from build123d import *

# Parameters (mm, degrees)
EXTRUDE_2_DEPTH     = 34.78
CUT_EXTRUDE_1_REACH = 62.522
SKETCH_2_W          = 20
SKETCH_2_H          = 20
CHAMFER_1_SIZE      = 1
CUT_EXTRUDE_START   = -34.54
SKETCH_3_R          = 2
CUT_EXTRUDE_2_DEPTH = 34.54
SKETCH_4_R          = 2
CUT_EXTRUDE_3_DEPTH = 5
EXTRUDE_START       = -2
EXTRUDE_3_DEPTH     = 5


with BuildPart() as part:
    # 草图1 → 凸台-拉伸2 (new body)
    with BuildSketch(Plane.XY):
        Polygon((0, 0), (0, 35.5), (5, 35.5), (5, 5), (29.54, 5), (29.54, 35.5), (34.54, 35.5), (34.54, 0), align=None)
    extrude(amount=EXTRUDE_2_DEPTH)

    # 切除-拉伸1: up to this face of the body (flat: up to its plane)
    cut_extrude_1_end = Plane(part.part.faces().sort_by_distance((0, 17.75, 17.39))[0])
    # 草图2 → 切除-拉伸1 (cut, up to the picked face)
    with BuildSketch(Plane(origin=(34.54, 0, 0), x_dir=(0, 0, -1), z_dir=(1, 0, 0)), mode=Mode.PRIVATE) as cut_extrude_1_sk1:
        with Locations((-17.28, 15)):
            Rectangle(SKETCH_2_W, SKETCH_2_H)
    cut_extrude_1_tool1 = split(extrude(cut_extrude_1_sk1.sketch, amount=-CUT_EXTRUDE_1_REACH, mode=Mode.PRIVATE), bisect_by=cut_extrude_1_end, keep=Keep.BOTH, mode=Mode.PRIVATE)
    add(cut_extrude_1_tool1.solids().sort_by(Axis((34.54, 15, 17.28), (-1, 0, 0)))[0], mode=Mode.SUBTRACT)

    # 倒角1
    chamfer_1_edges = [part.edges().sort_by_distance(p)[0] for p in [
        (34.54, 17.75, 0),
        (17.27, 0, 0),
        (0, 0, 17.39),
        (34.54, 35.5, 17.39),
        (34.54, 0, 17.39),
        (0, 17.75, 34.78),
        (17.27, 0, 34.78),
        (0, 17.75, 0),
        (34.54, 17.75, 34.78),
    ]]
    chamfer(chamfer_1_edges, length=CHAMFER_1_SIZE)

    # 草图3 → 切除-拉伸2 (cut)
    with BuildSketch(Plane(origin=(34.54, 0, 0), x_dir=(0, 0, -1), z_dir=(1, 0, 0)).offset(CUT_EXTRUDE_START)):
        with Locations((-30.53, 19.5)):
            Circle(SKETCH_3_R)
        with Locations((-4.25, 19.5)):
            Circle(SKETCH_3_R)
        with Locations((-4.25, 29.5)):
            Circle(SKETCH_3_R)
        with BuildLine():
            ThreePointArc((-31.619976701, 31.176887233), (-32.53, 29.5), (-31.619976701, 27.823112767))
            Line((-31.619976701, 27.823112767), (-30.53, 29.5))
            Line((-30.53, 29.5), (-31.619976701, 31.176887233))
        make_face()
        with BuildLine():
            Line((-30.53, 29.5), (-31.619976701, 27.823112767))
            ThreePointArc((-31.619976701, 27.823112767), (-30.53, 27.5), (-29.440023299, 27.823112767))
            Line((-29.440023299, 27.823112767), (-30.53, 29.5))
        make_face()
        with BuildLine():
            Line((-30.53, 29.5), (-29.440023299, 27.823112767))
            ThreePointArc((-29.440023299, 27.823112767), (-28.772167044, 28.546048587), (-28.53, 29.5))
            ThreePointArc((-28.53, 29.5), (-28.772167044, 30.453951413), (-29.440023299, 31.176887233))
            Line((-29.440023299, 31.176887233), (-30.53, 29.5))
        make_face()
        with BuildLine():
            ThreePointArc((-29.440023299, 31.176887233), (-30.53, 31.5), (-31.619976701, 31.176887233))
            Line((-31.619976701, 31.176887233), (-30.53, 29.5))
            Line((-30.53, 29.5), (-29.440023299, 31.176887233))
        make_face()
    extrude(amount=CUT_EXTRUDE_2_DEPTH, mode=Mode.SUBTRACT)

    # 草图4 → 切除-拉伸3 (cut)
    with BuildSketch(Plane.XZ):
        with Locations(Location((9.27, 27.39, 0), (0, 0, 270))):
            Circle(SKETCH_4_R)
        with Locations(Location((25.27, 27.39, 0), (0, 0, 270))):
            Circle(SKETCH_4_R)
        with Locations(Location((25.27, 7.39, 0), (0, 0, 270))):
            Circle(SKETCH_4_R)
        with Locations(Location((9.27, 7.39, 0), (0, 0, 270))):
            Circle(SKETCH_4_R)
    extrude(amount=-CUT_EXTRUDE_3_DEPTH, mode=Mode.SUBTRACT)

    # 草图8 → 凸台-拉伸3 (add)
    with BuildSketch(Plane.XY.offset(34.78).offset(EXTRUDE_START)):
        Polygon((1, 35.5), (1, 1), (33.54, 1), (33.54, 35.5), (29.54, 35.5), (29.54, 5), (5, 5), (5, 35.5), align=None)
        Polygon((34.54, 1), (34.54, 34.5), (34.54, 35.5), (33.54, 35.5), (33.54, 1), (1, 1), (1, 35.5), (0, 35.5), (0, 1), (0, 0), (1, 0), (33.54, 0), (34.54, 0), align=None)
    extrude_3 = extrude(amount=EXTRUDE_3_DEPTH)

    # 镜向1: 凸台-拉伸3 across plane
    add(extrude_3.mirror(Plane.XY.offset(17.39)))


solid = part.part
Source: CAD feature listing. Evaluate the final solid. Frame: model axes, mm. A direction names the side the tool comes from. Give positions to 0.01 mm unless a question says otherwise; leave off trailing zeros. Write each loop counter-clockwise with the first axis right and the second up, starting at its lowest first coordinate (ties: lowest second). Pieces come first, ordered by that corner, then holes. Notation, with made-up numbers: M 28.25,-40 L 41.25,-40 A24 ccw 41.25,-21 Z; hole C 63,-34 d11. An arc over 180 degrees is marked long. Return JSON: item names as keys, results as strings. Group by question number.
1) Cut plane A-A, the plane y = 12.5. Output: boundary loops of the cut face in (x, z), plus the area to 3 significant figures.
2) Set-up query: faces 4 (the face through (34.3, 35.2, 2)), 5 (the face through (5, 27, 17)), 6 (the face through (3, 15, 27.28)), 7 (the face through (34.05, 0.51, 17.17)). Return all of +Z, -Z, +X, -X, +Y, -Y with unobstructed straight access to the full face (end or side cutting, diameter ignored); none if empty.
3) Pull-direction query (X, two-part tool) for faces 1 (the face through (0.3, 0.3, 2)), 2 (the face through (34.03, 35.01, 17.17)), 3 (the face through (18, 5, 18)); classes: pulls with the +X half, pulls with the -X half, needs draft (parallel to the pull), parting line crosses it, or undercut.
4) Cut plane B-B, the plane z = 4.25. Output: boundary loops of the cut face in (x, y), plus the area to 3 significant figures.
5) Cut plane C-C, the plane x = 25.27. Output: boundary loops of the cut face in (y, z), plus the area to 3 significant figures.
6) Cut plane D-D, the plane z = 14.5. Output: boundary loops of the cut face in (x, y), plus the area to 3 significant figures.
7) Material intervals for line 1 along Y through (x, z) = (31.45, 4.25); line 2 along Z through (x, y) = (3.25, 29.5); line 3 along X through (y, z) = (34, 27), sorted ascending. Write a range as [from, to].
Recorded:
{
 "1": {"outline": "M 0,-3 L 5,-3 L 5,7.28 L 0,7.28 Z; M 0,27.28 L 5,27.28 L 5,37.78 L 0,37.78 Z; M 29.54,-3 L 34.54,-3 L 34.54,7.28 L 29.54,7.28 Z; M 29.54,27.28 L 34.54,27.28 L 34.54,37.78 L 29.54,37.78 Z", "area": "208 mm²"},
 "2": {"face 4": "+X, +Y", "face 5": "+Z, -Z, +Y", "face 6": "+X, -X", "face 7": "+X, -Y"},
 "3": {"face 1": "needs draft", "face 2": "pulls with the +X half", "face 3": "undercut"},
 "4": {"outline": "M 0,1 L 1,0 L 33.54,0 L 34.54,1 L 34.54,17.5 L 29.54,17.5 L 29.54,5 L 5,5 L 5,17.5 L 0,17.5 Z; M 0,21.5 L 5,21.5 L 5,27.5 L 0,27.5 Z; M 0,31.5 L 5,31.5 L 5,35.5 L 0,35.5 Z; M 29.54,21.5 L 34.54,21.5 L 34.54,27.5 L 29.54,27.5 Z; M 29.54,31.5 L 34.54,31.5 L 34.54,34.5 L 33.54,35.5 L 29.54,35.5 Z", "area": "396 mm²"},
 "5": {"outline": "M 0,-3 L 5,-3 L 5,5.39 L 0,5.39 Z; M 0,9.39 L 5,9.39 L 5,25.39 L 0,25.39 Z; M 0,29.39 L 5,29.39 L 5,37.78 L 0,37.78 Z", "area": "164 mm²"},
 "6": {"outline": "M 0,1 L 1,0 L 33.54,0 L 34.54,1 L 34.54,5 L 0,5 Z; M 0,25 L 5,25 L 5,35.5 L 0,35.5 Z; M 29.54,25 L 34.54,25 L 34.54,34.5 L 33.54,35.5 L 29.54,35.5 Z", "area": "276 mm²"},
 "7": {"line 1": "y = [0, 17.5], [21.5, 27.5], [31.5, 35.5]", "line 2": "z = [-3, 2.25], [6.25, 28.53], [32.53, 37.78]", "line 3": "x = [0, 5], [29.54, 34.54]"}
}
